```python
from build123d import *

# Parameters (mm, degrees)
F0_W     = 66.73024
F0_H     = 62.78385
F1_DEPTH = 25
F2_R     = 10.820762
F4_DEPTH = 25
F5_D     = 5


with BuildPart() as f1:
    # F0 (on Right) → F1 (new body)
    with BuildSketch(Plane.YZ):
        with Locations((-23.582063, 2.156687)):
            Rectangle(F0_W, F0_H)
    extrude(amount=F1_DEPTH)

    # F2 (on face) → F4 (join)
    with BuildSketch(Plane.YZ.offset(25)):
        with Locations((-27.518781, 9.579325)):
            Circle(F2_R)
    extrude(amount=-F4_DEPTH)

    # F5 (through all)
    with Locations(Plane.YZ.offset(25)):
        with Locations((-7.812866, 0)):
            Hole(F5_D / 2)


solid = f1.part
```
Read the model definition and answer for the solid it produces. Units are mm, in the model's axes. Coordinates: 2 decimals unless noted, no trailing zeros. Write each loop counter-clockwise with the first axis right and the second up, starting at its lowest first coordinate (ties: lowest second). Pieces come first, ordered by that corner, then holes. Notation, with made-up numbers: (-22.5, 14.25) -> (-0.5, 14.25) arc R12 ccw to (-0.5, 27.25) -> close; hole circle Ø2 at (8.5, 12). An arc over 180 degrees is marked (long way). Return JSON: item names as keys, results as strings.
1. A cutting plane is placed at A-A (z = 0). Determine the outline of the cut face in (x, y).
Found:
{"outline": "(0, -56.95) -> (25, -56.95) -> (25, -10.31) -> (0, -10.31) -> close; (0, -5.31) -> (25, -5.31) -> (25, 9.78) -> (0, 9.78) -> close"}
2. Determine the mould class of faces 1 (the face through (12, -24, -29.235)), 2 (the face through (25, -24, 3)), 3 (the face through (12.325, -5.315, 0.11)) for opening direction Z: pulls with the +Z half, pulls with the -Z half, needs draft (parallel to the pull), parting line crosses it, or undercut.
Found:
{"face 1": "pulls with the -Z half", "face 2": "needs draft", "face 3": "undercut"}
3. Find the intervals of material crossed by line 1 along Y through (x, z) = (1, -2); line 2 along Z through (x, y) = (2, -9.5); line 3 along Y through (x, z) = (22.5, -1), in increasing order. Write a range as from..to.
Found:
{"line 1": "-56.95..-9.31, -6.31..9.78", "line 2": "-29.24..-1.84, 1.84..33.55", "line 3": "-56.95..-10.1, -5.52..9.78"}
